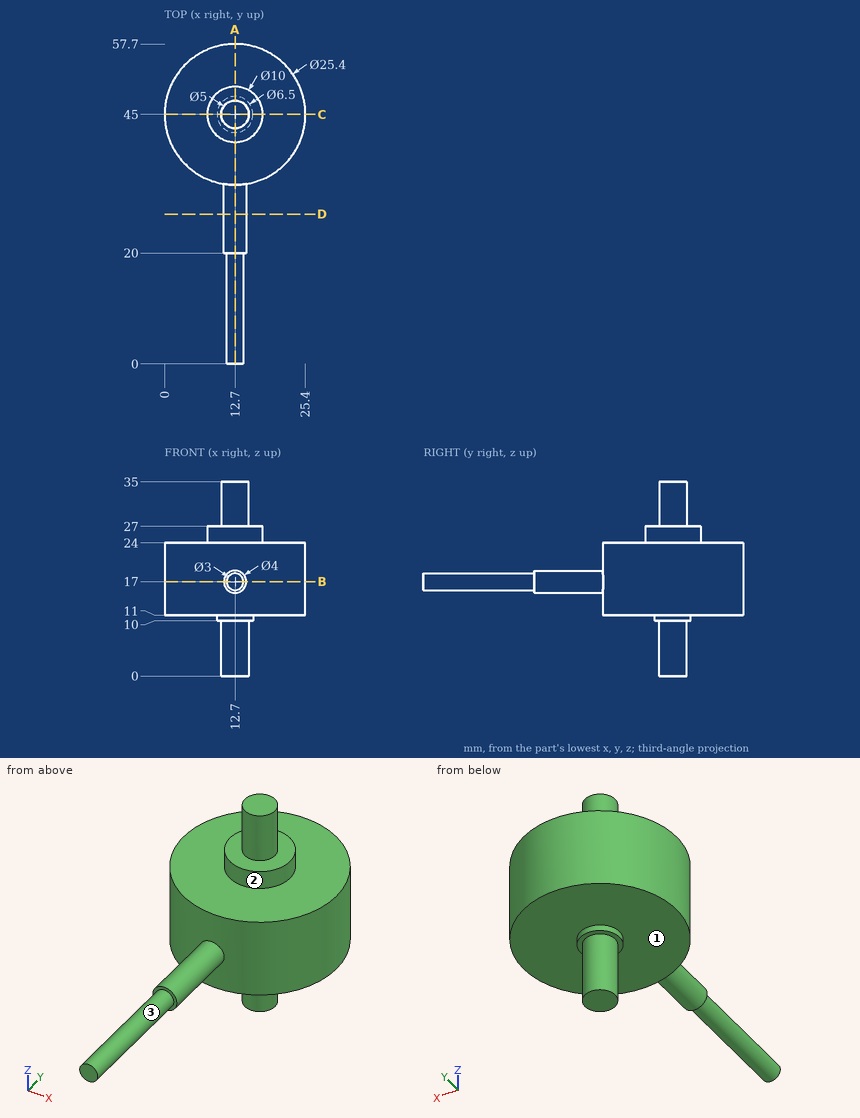
Study the drawing (mm; zero at the part's minimum x, y, z) and answer. A direction names the side the tool comes from. Round coordinates to 2 decimals unless told otherwise and drop trailing zeros. Write each loop counter-clockwise with the first axis right and the second up, starting at its lowest first coordinate (ties: lowest second). Pieces come first, ordered by that corner, then holes.
1) A cutting plane is placed at D-D (y = 27). Give the vertices of the cut face in (x, z).
2) A cutting plane is placed at A-A (x = 12.7). Give the vertices of the cut face in (y, z).
3) A cutting plane is placed at C-C (y = 45). Give the vertices of the cut face in (x, z), plus the area to 3 significant figures.
4) A cutting plane is placed at B-B (z = 17). Give the vertices of the cut face in (x, y), plus the area to 3 significant figures.
5) Given pin 1 Ø2 at (x, z) = (14.5, 14) entering from +Y; pin 2 Ø10 at (x, z) = (8, 7) entering from +Y; pin 3 Ø2 at (y, z) = (49, 17) entering from +X, each flat-ended and moving along its own axis, determine where each tip first touches the part or whether it passes through.
6) Straight lines are drawn through the part: line 1 (Z direction, x = 15.75, y = 37); line 2 (Y direction, x = 22.25, z = 20); line 3 (Y direction, x = 12, z = 28.5). For each, find the intervals that lie inside material, in ascending order.
7) A tool of negligible diameter and unlimited length cuts with its end or side. For the marked faces 1, 2 and 3, from which of +Z, -Z, +X, -X, +Y, -Y can it reach the whole face along a straight path? Write none if from no direction.
Completed:
1. outline: circle Ø4 at (12.7, 17)
2. outline: (0, 15.5) - (20, 15.5) - (20, 15) - (32.3, 15) - (32.3, 11) - (41.75, 11) - (41.75, 10) - (42.5, 10) - (42.5, 0) - (47.5, 0) - (47.5, 10) - (48.25, 10) - (48.25, 11) - (57.7, 11) - (57.7, 24) - (50, 24) - (50, 27) - (47.5, 27) - (47.5, 35) - (42.5, 35) - (42.5, 27) - (40, 27) - (40, 24) - (32.3, 24) - (32.3, 19) - (20, 19) - (20, 18.5) - (0, 18.5) - close
3. outline: (0, 11) - (9.45, 11) - (9.45, 10) - (10.2, 10) - (10.2, 0) - (15.2, 0) - (15.2, 10) - (15.95, 10) - (15.95, 11) - (25.4, 11) - (25.4, 24) - (17.7, 24) - (17.7, 27) - (15.2, 27) - (15.2, 35) - (10.2, 35) - (10.2, 27) - (7.7, 27) - (7.7, 24) - (0, 24) - close
3. area: 457 mm2
4. outline: (10.7, 20) - (11.2, 20) - (11.2, 0) - (14.2, 0) - (14.2, 20) - (14.7, 20) - (14.7, 32.46) arc R12.7 ccw (long way) to (10.7, 32.46) - close
4. area: 616 mm2
5. pin 1: stops at y = 57.67
5. pin 2: stops at y = 57.59
5. pin 3: stops at x = 25.04
6. line 1: z = 11 to 24
6. line 2: y = 36.63 to 53.37
6. line 3: y = 42.6 to 47.4
7. face 1: -Z
7. face 2: +Z
7. face 3: -Y
